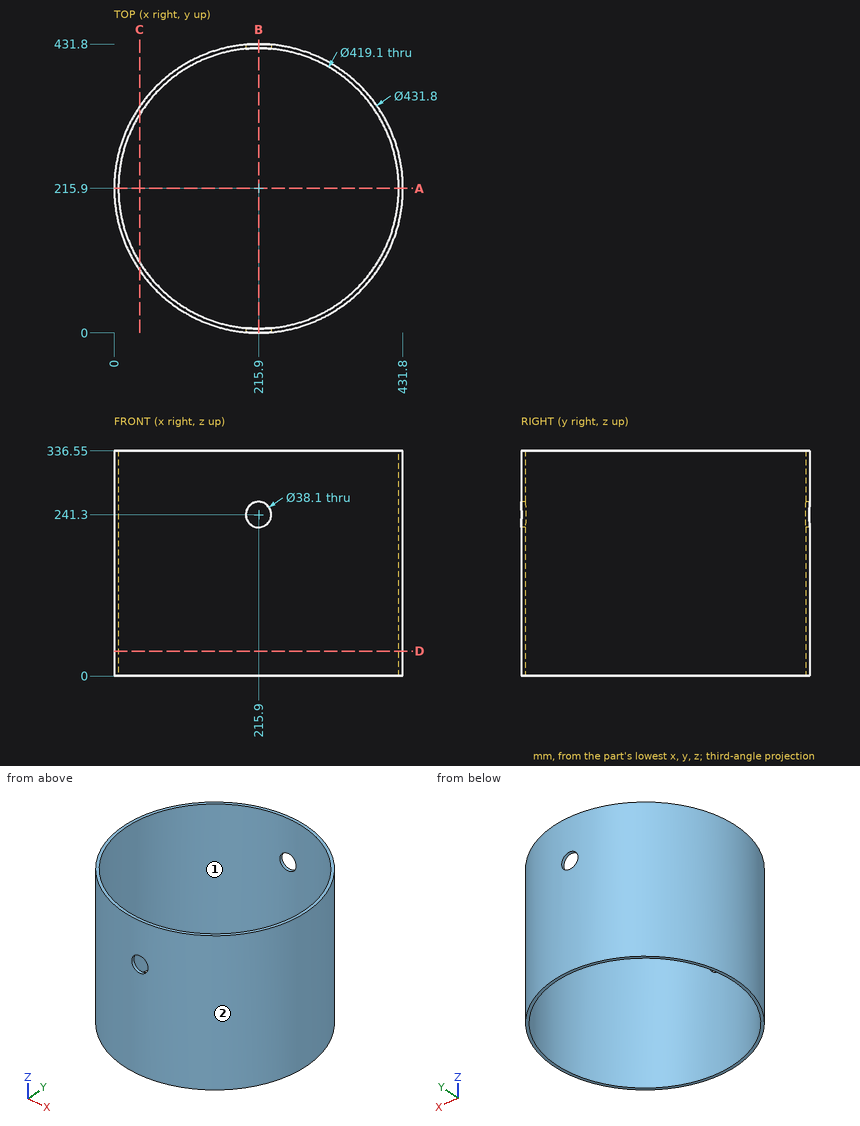
Here's the drawing with two shaded views (mm, measured from the low corner). I have some questions. Coordinates: 2 decimals unless noted, no trailing zeros. Order: outer loops, then holes, each group sorted by start corner. A loop starts at its lowest first (then second) coordinate and runs counter-clockwise, first axis right, second up.
Q1. Suppose I cut it at B-B on x = 215.9. Please give me the cut outline in (y, z).
Q2. Suppose I cut it at C-C on x = 38. Please give me the cut outline in (y, z), and give its area (3 significant figures).
Q3. Please list where these lines run through material, in increasing order: L1, parallel to Y at x = 222.5, z = 304; L2, parallel to Z at x = 215.9, y = 430.25; L3, parallel to X at y = 215, z = 149.
Q4. Thinking about a two-plate mould opening in X: for the marked faces 1 and 2, which applies, released by +X, released by -X, zero draft, split by the parting line, or undercut?
Q5. Suppose I cut it at A-A on y = 215.9. Please give me the cut outline in (x, z).
Q6. Suppose I cut it at D-D on z = 37. Please give me the cut outline in (x, y), and give its area (3 significant figures).
Q7. Will these pins go through, and if not, where does the flat tip stop? pin 1 (10 mm diameter, centred on x = 329.5, z = 50.5, fed in from +Y); pin 2 (1.5 mm diameter, centred on y = 257.5, z = 237.5, fed in from -X); pin 3 (4 mm diameter, centred on y = 247, z = 163, fed in from +X).
Answer:
1. outline: (0, 0) - (6.35, 0) - (6.35, 222.25) - (0, 222.25) - close; (0, 260.35) - (6.35, 260.35) - (6.35, 336.55) - (0, 336.55) - close; (425.45, 0) - (431.8, 0) - (431.8, 222.25) - (425.45, 222.25) - close; (425.45, 260.35) - (431.8, 260.35) - (431.8, 336.55) - (425.45, 336.55) - close
2. outline: (93.57, 0) - (105.16, 0) - (105.16, 336.55) - (93.57, 336.55) - close; (326.64, 0) - (338.23, 0) - (338.23, 336.55) - (326.64, 336.55) - close
2. area: 7,800 mm2
3. L1: y = 0.1 to 6.45, 425.35 to 431.7
3. L2: z = 0 to 222.25, 260.35 to 336.55
3. L3: x = 0 to 6.35, 425.45 to 431.8
4. face 1: undercut
4. face 2: split by the parting line
5. outline: (0, 0) - (6.35, 0) - (6.35, 336.55) - (0, 336.55) - close; (425.45, 0) - (431.8, 0) - (431.8, 336.55) - (425.45, 336.55) - close
6. outline: circle Ø431.8 at (215.9, 215.9); hole circle Ø419.1 at (215.9, 215.9)
6. area: 8,490 mm2
7. pin 1: stops at y = 402.5
7. pin 2: stops at x = 3.9
7. pin 3: stops at x = 429.83
